Check sheet for the modelled part. Datum: model origin and axes. Units: mm. Face numbers are marked on the shaded views. A direction names the side the tool comes from. Coordinates: 2 decimals unless noted, no trailing zeros. Write each loop counter-clockwise with the first axis right and the second up, starting at its lowest first coordinate (ties: lowest second). Pieces come first, ordered by that corner, then holes. Notation, with made-up numbers: M 49,49.5 L 76,49.5 A7 cw 76,53.5 Z; hole C 79.5,39 d9. An arc over 180 degrees is marked long. Answer as CSV lines item,"result".
from build123d import *

# Parameters (mm, degrees)
F0_W     = 25
F0_H     = 25
F1_DEPTH = 2
F3_DEPTH = 25
F4_W     = 5
F4_H     = 2.2
F4_R     = 3
F5_DEPTH = 2
F6_R     = 1.8
F7_DEPTH = 18.280056
F9_DEPTH = 4


with BuildPart() as f1:
    # F0 (on Top) → F1 (new body)
    with BuildSketch(Plane.XY):
        Rectangle(F0_W, F0_H)
    extrude(amount=F1_DEPTH)

    # F2 (on face) → F3 (join, through all)
    with BuildSketch(Plane(origin=(-12.5, 0, 0), x_dir=(0, -1, 0), z_dir=(-1, 0, 0))):
        Polygon((-12.5, 16.279056), (-12.5, 2), (-8.5, 2), (-8.5, 12.237604), (-7.5, 12.237604), (8.5, 3), (8.5, 2), (12.5, 2), (12.5, 5.309401), (-6.5, 16.279056), align=None)
    extrude(amount=-F3_DEPTH)

    # F4 (on face) → F5 (join)
    with BuildSketch(Plane(origin=(0, 0, 0), x_dir=(1, 0, 0), z_dir=(0, 0, -1))):
        with Locations((0, -8.9)):
            Rectangle(F4_W, F4_H)
        with Locations((0, 5.95)):
            Circle(F4_R)
    extrude(amount=F5_DEPTH)

    # F6 (on face) → F7 (cut, through all)
    with BuildSketch(Plane(origin=(0, 0, -2), x_dir=(1, 0, 0), z_dir=(0, 0, -1))):
        with Locations((0, 5.95)):
            Circle(F6_R)
    extrude(amount=-F7_DEPTH, mode=Mode.SUBTRACT)

    # F8 (on face) → F9 (cut, through all)
    with BuildSketch(Plane(origin=(0, 12.5, 0), x_dir=(-1, 0, 0), z_dir=(0, 1, 0))):
        Polygon((2.375, 4.025907), (4.75, 8.139528), (2.375, 12.253149), (-2.375, 12.253149), (-4.75, 8.139528), (-2.375, 4.025907), align=None)
    extrude(amount=-F9_DEPTH, mode=Mode.SUBTRACT)


solid = f1.part
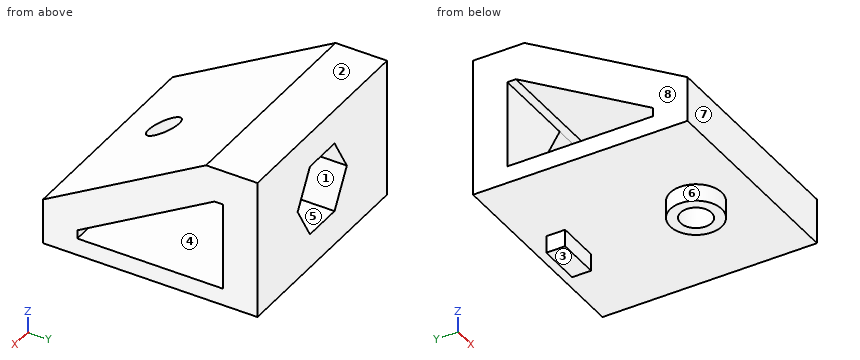
1) Section check B-B, the plane x = -7.5. Record the boundary of the cut face in (y, z).
Answer key:
outline,"M -12.5,0 L 12.5,0 L 12.5,16.28 L 6.5,16.28 L -12.5,5.31 Z; hole M -8.5,2 L 8.5,2 L 8.5,12.24 L 7.5,12.24 L -8.5,3 Z"
2) Depth check by flat-ended pin: P1, Ø13.5, axis at x = 3, y = 2.5, coming from the +Z side; P2, Ø3, axis at x = 0, y = -5.95, coming from the +Z side; P3, Ø8, axis at x = 8.5, y = 8, coming from the -Z side; P4, Ø1.6, axis at y = 8.5, z = -1.5, coming from the -X side. Enter the tip coordinate at first touch or a pass-through.
Answer key:
P1,"stops at z = 16.28"
P2,"passes through"
P3,"stops at z = 0"
P4,"stops at x = -2.5"
3) Thickness scan on line 1 along Y through (x, z) = (0, -0.6); line 2 along Z through (x, y) = (3.25, 8.25); line 3 along X through (y, z) = (-5.95, 1.1). Record the ranges inside material, lowest first.
Answer key:
line 1,"y = -8.95 to -7.75, -4.15 to -2.95, 7.8 to 10"
line 2,"z = 0 to 2, 12.24 to 16.28"
line 3,"x = -12.5 to -1.8, 1.8 to 12.5"
4) Section check C-C, the plane y = -6.5. Record the boundary of the cut face in (x, z).
Answer key:
outline,"M -12.5,0 L -2.95,0 L -2.95,-2 L -1.71,-2 L -1.71,2 L -12.5,2 Z; M -12.5,4.15 L -1.71,4.15 L -1.71,8.77 L -12.5,8.77 Z; M 1.71,-2 L 2.95,-2 L 2.95,0 L 12.5,0 L 12.5,2 L 1.71,2 Z; M 1.71,4.15 L 12.5,4.15 L 12.5,8.77 L 1.71,8.77 Z"
5) Section check A-A, the plane y = 7. Record the boundary of the cut face in (x, z).
Answer key:
outline,"M -12.5,0 L 12.5,0 L 12.5,2 L -12.5,2 Z; M -12.5,11.95 L 12.5,11.95 L 12.5,16.28 L -12.5,16.28 Z"
6) Tool access check on the marked faces 4, 5, 6, 7 and 8. Record the directions out of +Z, -Z, +X, -X, +Y, -Y that give a thin tool (end or side, any length) a straight path to the whole face; none if there is none.
Answer key:
face 4,"+X, -X"
face 5,"+Y"
face 6,"-Z"
face 7,"+Z, -Z, +X, -X, -Y"
face 8,"+Z, -Z, -X, +Y, -Y"
7) Mould release check, pull along Z, two halves, no side actions. Record for the marked faces 1, 2 and 3: pulls with the +Z half, pulls with the -Z half, needs draft (parallel to the pull), parting line crosses it, or undercut.
Answer key:
face 1,"undercut"
face 2,"pulls with the +Z half"
face 3,"pulls with the -Z half"
8) Section check D-D, the plane x = 0. Give the number of separate pieces and of enclosed holes in the cut face, plus the area to 3 significant figures.
Answer key:
separate pieces,"3"
enclosed holes,"0"
area,"155 mm2"
